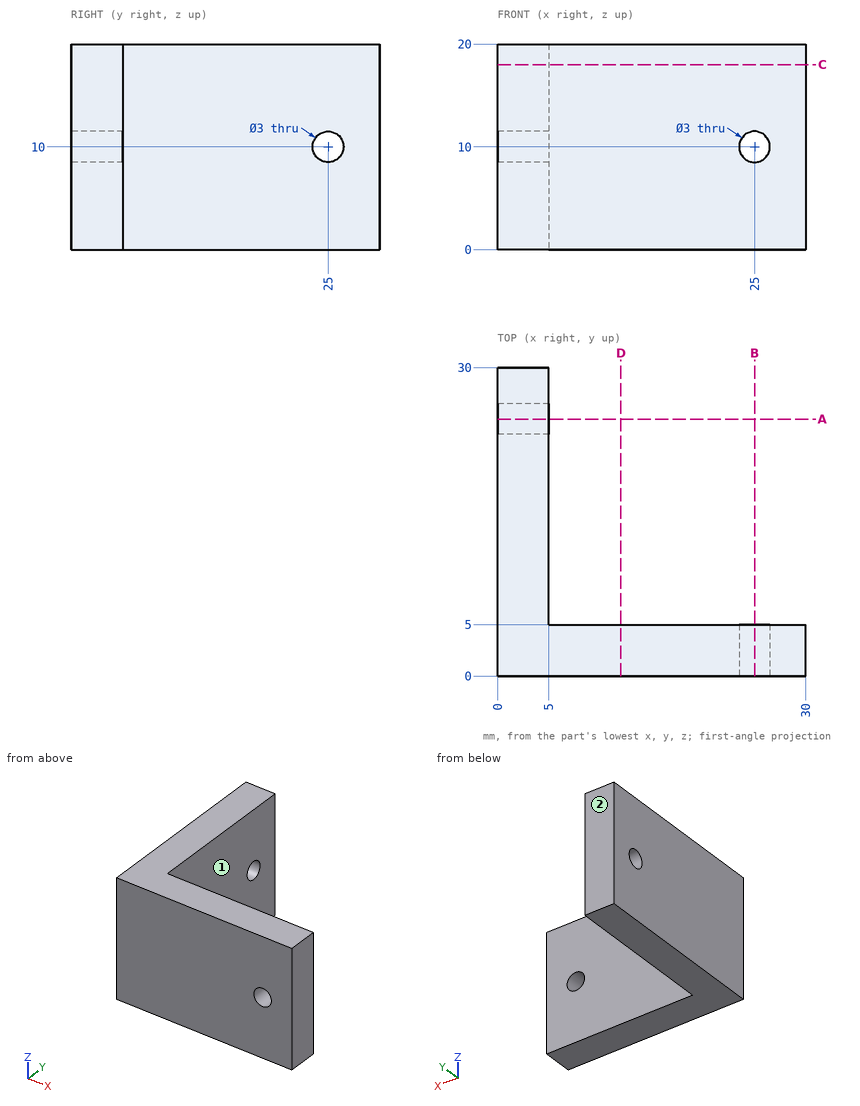
Can you work these out from the drawing? Everything is in mm from the part's minimum corner. A direction names the side the tool comes from. Round coordinates to 2 decimals unless told otherwise and drop trailing zeros. Order: outer loops, then holes, each group sorted by start corner. A loop starts at its lowest first (then second) coordinate and runs counter-clockwise, first axis right, second up. Notation, with made-up numbers: (33.25, -4.75) - (56.25, -4.75) arc R19 cw to (56.25, 30.25) - close; hole circle Ø4 at (84, -23.5). An arc over 180 degrees is marked (long way). Answer in a Markdown table with one row per item.
(1) Please list where these lines run through material, in increasing order: L1, parallel to Z at x = 25, y = 2.75; L2, parallel to X at y = 3.2, z = 10. Write a range as from..to.
From the geometry:
| item | result |
|---|---|
| L1 | z = 0..8.5, 11.5..20 |
| L2 | x = 0..23.5, 26.5..30 |
(2) Suppose I cut it at C-C, the plane z = 18. Please give me the cut outline in (x, y), plus the area to 3 significant figures.
From the geometry:
| item | result |
|---|---|
| outline | (0, 0) - (30, 0) - (30, 5) - (5, 5) - (5, 30) - (0, 30) - close |
| area | 275 mm2 |
(3) Suppose I cut it at A-A, the plane y = 25. Please give me the cut outline in (x, z), plus the area to 3 significant figures.
From the geometry:
| item | result |
|---|---|
| outline | (0, 0) - (5, 0) - (5, 8.5) - (0, 8.5) - close; (0, 11.5) - (5, 11.5) - (5, 20) - (0, 20) - close |
| area | 85.0 mm2 |
(4) Suppose I cut it at D-D, the plane x = 12. Please give me the cut outline in (y, z), plus the area to 3 significant figures.
From the geometry:
| item | result |
|---|---|
| outline | (0, 0) - (5, 0) - (5, 20) - (0, 20) - close |
| area | 100 mm2 |
(5) For P1, Ø10, axis at x = 12.5, z = 6.5, coming from the +Y side; P2, Ø2.5, axis at y = 25, z = 10, coming from the +X side, each with a flat end and sliding along its axis, tell me the tip position at first contact or that it passes through.
From the geometry:
| item | result |
|---|---|
| P1 | stops at y = 5 |
| P2 | passes through |
(6) Which directions (+Z, -Z, +X, -X, +Y, -Y) give clear straight access to the entire face, cutting with the end or side of a thin tool? Please do the marked faces 1 and 2.
From the geometry:
| item | result |
|---|---|
| face 1 | +Z, -Z, +X, +Y |
| face 2 | +Z, -Z, +X, -X, +Y |
